The drawing under review shows one solid part. Ordinate dimensions are in mm from its lowest x, y, z. A direction names the side the tool comes from. Coordinates: 2 decimals unless noted, no trailing zeros. Order: outer loops, then holes, each group sorted by start corner. A loop starts at its lowest first (then second) coordinate and runs counter-clockwise, first axis right, second up. Notation, with made-up numbers: (-16.75, -20.75) - (24.25, -20.75) arc R27 ccw to (24.25, 12.25) - close; hole circle Ø10 at (6.5, 44.25). An arc over 180 degrees is marked (long way). Answer in a Markdown table with one row per item.
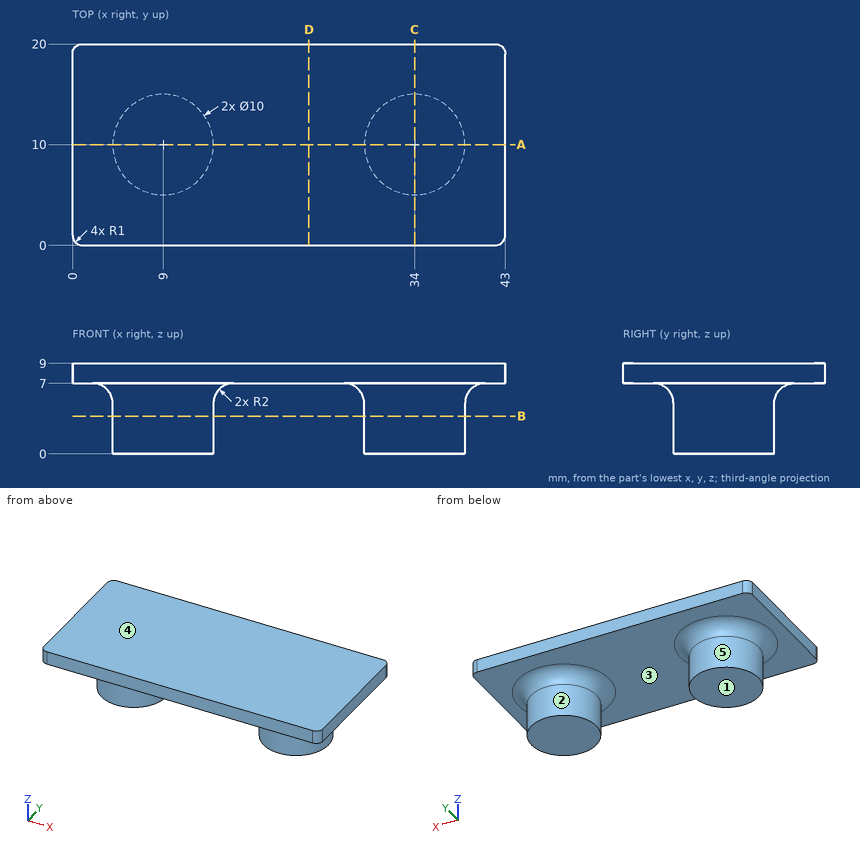
Item 1: We need section B-B, the plane z = 3.75. Write out the cut boundary in (x, y), then the cut area to 3 significant figures.
Check values:
| item | result |
|---|---|
| outline | circle Ø10 at (9, 10); circle Ø10 at (34, 10) |
| area | 157 mm^2 |
Item 2: Mouldability with a two-part tool opening along Z and no side actions: class the marked faces 3, 4 and 5 as +Z half, -Z half, draft (parallel to the pull), parting line (faces both ways), or undercut.
Check values:
| item | result |
|---|---|
| face 3 | -Z half |
| face 4 | +Z half |
| face 5 | draft |
Item 3: To check wall thickness, follow line 1 (Z direction, x = 25, y = 17.5); line 2 (X direction, y = 12, z = 2.5); line 3 (X direction, y = 14, z = 4.75). State the ranges of each line that lie inside material, in increasing order. Write a range as from..to.
Check values:
| item | result |
|---|---|
| line 1 | 7..9 |
| line 2 | 4.42..13.58, 29.42..38.58 |
| line 3 | 6..12, 31..37 |
Item 4: Clearance check with flat-ended pins moving along their axes: pin 1 Ø1 at (y, z) = (12, 5) entering from +X; pin 2 Ø5 at (x, z) = (14, 8) entering from -Y. State where each tip first meets the part, or that it passes through.
Check values:
| item | result |
|---|---|
| pin 1 | x = 38.77 |
| pin 2 | y = 0 |
Item 5: We need section D-D, the plane x = 23.5. Write out the cut boundary in (y, z).
Check values:
| item | result |
|---|---|
| outline | (0, 7) - (20, 7) - (20, 9) - (0, 9) - close |
Item 6: We need section A-A, the plane y = 10. Write out the cut boundary in (x, z), then the cut area to 3 significant figures.
Check values:
| item | result |
|---|---|
| outline | (0, 7) - (2, 7) arc R2 cw to (4, 5) - (4, 0) - (14, 0) - (14, 5) arc R2 cw to (16, 7) - (27, 7) arc R2 cw to (29, 5) - (29, 0) - (39, 0) - (39, 5) arc R2 cw to (41, 7) - (43, 7) - (43, 9) - (0, 9) - close |
| area | 229 mm^2 |
Item 7: Tool access review of the marked faces 1 and 2: name each direction out of +Z, -Z, +X, -X, +Y, -Y from which nothing blocks a thin tool from reaching the whole face with its end or side.
Check values:
| item | result |
|---|---|
| face 1 | -Z, +X, -X, +Y, -Y |
| face 2 | -Z |
Item 8: We need section C-C, the plane x = 34. Write out the cut boundary in (y, z), then the cut area to 3 significant figures.
Check values:
| item | result |
|---|---|
| outline | (0, 7) - (3, 7) arc R2 cw to (5, 5) - (5, 0) - (15, 0) - (15, 5) arc R2 cw to (17, 7) - (20, 7) - (20, 9) - (0, 9) - close |
| area | 112 mm^2 |
